Autodesk Fusion 360 part; units mm, degrees
sketch "Sketch1" plane through (0, 0, 0) normal (0, 0, 1) x (1, 0, 0)
  line L0 (0, 0) -> (76, 0)
  line L1 (76, 0) -> (76, 76)
  line L2 (76, 76) -> (0, 76)
  line L3 (0, 76) -> (0, 0)
  dimension "d1" = 76
  dimension "d2" = 76
extrude "Extrude1" add sketch "Sketch1" along normal blind 6.35
sketch "Sketch2" plane through (0, 0, 6.35) normal (0, 0, 1) x (-1, 0, 0)
  line L0 (0, -76) -> (0, 0)
  line L1 (0, 0) -> (-76, 0)
  line L2 (-76, 0) -> (-76, -76)
  line L3 (-76, -76) -> (0, -76)
  line L4 (-52, -66) -> (-38, -66)
  line L5 (-38, -66) -> (-38, -91)
  line L6 (-38, -91) -> (-52, -91)
  line L7 (-52, -91) -> (-52, -66)
  dimension "d5" = 14
  dimension "d6" = 25
  dimension "d7" = 24
  dimension "d8" = 10
extrude "Extrude2" add sketch "Sketch2" along normal blind 10 contours L3 L5 L6 L7 | L3 L4 L5 L7
fillet "Fillet1" radius 10 1 edges at (45, 66, 16.35)
fillet "Fillet2" radius 5 2 edges at (45, 91, 16.35) (45, 91, 6.35)
sketch "Sketch3" plane through (0, 0, 16.35) normal (0, 0, 1) x (-1, 0, 0)
  line L0 (-52, -86) -> (-38, -86)
  line L1 (-38, -86) -> (-38, -76)
  line L2 (-38, -76) -> (-52, -76)
  line L3 (-52, -76) -> (-52, -86)
  line L4 (-50, -80) -> (-40, -80)
  line L5 (-40, -80) -> (-40, -95)
  line L6 (-40, -95) -> (-50, -95)
  line L7 (-50, -95) -> (-50, -80)
extrude "Extrude3" cut sketch "Sketch3" against normal blind 20 contours L0 L4 L5 L7 | L0 L5 L6 L7
sketch "Sketch4" plane through (40, 0, 0) normal (1, 0, 0) x (0, 1, 0)
  line L0 (80, 6.35) -> (86, 6.35)
  arc A0 (86, 6.35) -> (86, 16.35) centre (86, 11.35) ccw
  line L1 (86, 16.35) -> (80, 16.35)
  line L2 (80, 16.35) -> (80, 6.35)
  circle A1 centre (86, 11.35) radius 3.25
  dimension "d17" = 6.5
extrude "Extrude4" add sketch "Sketch4" along normal blind 10 contours A1
extrude "Extrude5" add 1 faces at (76, 25.3333, 2.1167) along direction (1, 0, 0) blind 5
extrude "Extrude6" add 1 faces at (0, 50.6667, 2.1167) along direction (-1, 0, 0) blind 5
extrude "Extrude7" add 1 faces at (23.6667, 0, 2.1167) along direction (0, -1, 0) blind 5
sketch "Sketch5" plane through (0, 0, 6.35) normal (0, 0, 1) x (-1, 0, 0)
  line L0 (-38, -66) -> (-38, -76)
  line L1 (-38, -76) -> (5, -76)
  line L2 (5, -76) -> (5, 5)
  line L3 (5, 5) -> (-81, 5)
  line L4 (-81, 5) -> (-81, -76)
  line L5 (-81, -76) -> (-52, -76)
  line L6 (-52, -76) -> (-52, -66)
  line L7 (-52, -66) -> (-38, -66)
  line L8 (-81, -76) -> (-76.6575, -76)
  line L9 (-76.6575, -76) -> (-76.6575, -71)
  line L10 (-76.6575, -71) -> (-81, -71)
  line L11 (-81, -71) -> (-81, -76)
  line L12 (5, -76) -> (0, -76)
  line L13 (0, -76) -> (0, -71)
  line L14 (0, -71) -> (5, -71)
  line L15 (5, -71) -> (5, -76)
  line L16 (5, 5) -> (0, 5)
  line L17 (0, 5) -> (0, 0)
  line L18 (0, 0) -> (5, 0)
  line L19 (5, 0) -> (5, 5)
  line L20 (-81, 5) -> (-76, 5)
  line L21 (-76, 5) -> (-76, 0)
  line L22 (-76, 0) -> (-81, 0)
  line L23 (-81, 0) -> (-81, 5)
  dimension "d26" = 5
  dimension "d27" = 5
  dimension "d28" = 5
  dimension "d29" = 5
  dimension "d30" = 5
  dimension "d31" = 5
  dimension "d32" = 5
extrude "Extrude8" add sketch "Sketch5" along normal blind 25 contours L1 L2 L12 L13 L14 L15 | L4 L5 L8 L9 L10 L11 | L2 L3 L16 L17 L18 L19 | L3 L4 L20 L21 L22 L23
Check sheet for the modelled part. Datum: model origin and axes. Units: mm. A direction names the side the tool comes from. Give positions to 0.01 mm unless a question says otherwise; leave off trailing zeros. Order: outer loops, then holes, each group sorted by start corner. A loop starts at its lowest first (then second) coordinate and runs counter-clockwise, first axis right, second up. Notation, with made-up numbers: (81.25, 58) - (127.25, 58) arc R23 cw to (127.25, 90) - close; hole circle Ø7 at (69, 3). An arc over 180 degrees is marked (long way). Answer as CSV lines item,"result".
1. Section check B-B (z = 5). Record the boundary of the cut face in (x, y).
Result sheet:
outline,"(-5, -5) - (81, -5) - (81, 76) - (-5, 76) - close"
2. Mould release check, pull along X, two halves, no side actions. Record for faces 5 (the face through (52, 79, 11)), 6 (the face through (-5, 36, 6)), 7 (the face through (76, -3, 19)), 8 (the face through (51.01, 89.57, 14.85)): released by +X, released by -X, zero draft, split by the parting line, or undercut.
Result sheet:
face 5,"undercut"
face 6,"released by -X"
face 7,"undercut"
face 8,"zero draft"
3. Scan lines: probe 1 along Y at (x, z) = (-1, 10.5); probe 2 along X at (y, z) = (74, 20.5); probe 3 along Z at (x, y) = (3, 28.5). Record each from-to range of solid material in increasing order. Write a range as from..to.
Result sheet:
probe 1,"-5..0, 71..76"
probe 2,"-5..0, 76.66..81"
probe 3,"0..6.35"
4. Tool access check on faces 1 (the face through (78, 0, 19)), 2 (the face through (79, 71, 19)), 3 (the face through (0, 74, 19)), 4 (the face through (45, 79, 6.35)). Record the directions out of +Z, -Z, +X, -X, +Y, -Y that give a thin tool (end or side, any length) a straight path to the whole face; none if there is none.
Result sheet:
face 1,"+Z, +X, -X"
face 2,"+Z, +X"
face 3,"+Z, +Y, -Y"
face 4,"-Z, +X, -X, +Y"
5. Section check C-C (y = 54). Record the boundary of the cut face in (x, z).
Result sheet:
outline,"(-5, 0) - (81, 0) - (81, 6.35) - (-5, 6.35) - close"
6. Go/stop test with flat-tipped pins: P1, Ø3, axis at x = 26, y = 16.5, coming from the -Z side; P2, Ø3, axis at y = 80, z = 12.5, coming from the -X side; P3, Ø11, axis at x = 48.5, y = 78.5, coming from the +Z side; P4, Ø1.5, axis at x = -1.5, z = 21.5, coming from the +Y side. Record where each tip stops, or that it passes through.
Result sheet:
P1,"z = 0"
P2,"x = 38"
P3,"z = 16.35"
P4,"y = 76"
